Work out the finished part from the listing and answer in its coordinate system (mm). Face numbers are marked on the shaded views. A direction names the side the tool comes from. Give positions to 0.01 mm unless a question says otherwise; leave off trailing zeros. Loops run counter-clockwise (first coordinate to the right, second up) from the corner with the lowest first, then second, coordinate; pieces in that order, holes last.
from build123d import *

# Parameters (mm, degrees)
SHIM_TOP_START          = -1.6
SHIM_SKETCH_W           = 10.2
SHIM_SKETCH_H           = 2.6
SHIM_TOP_DEPTH          = 8.4
SHIM_BOTTOM_OUTLINE_W   = 10.027211308
SHIM_BOTTOM_OUTLINE_H   = 2.427211308
SHIM_BOTTOM_DEPTH       = 19.8
SHIM_BOTTOM_DRAFT       = -0.25
CHAMFER_2_SIZE          = 1
CHAMFER_2_SIZE2         = 1.745257156
RETAINING_BUMP_SKETCH_R = 3.5
RETAINING_BUMP_DEPTH    = 0.3
FILLET1_R               = 0.3


# Read off the part's stored shape, not the designer's step: shim_bottom
with BuildPart() as part:
    # shim_sketch → shim_top (new body)
    with BuildSketch(Plane.XY.offset(SHIM_TOP_START)):
        with Locations((-242.85, 41.3)):
            Rectangle(SHIM_SKETCH_W, SHIM_SKETCH_H)
    extrude(amount=-SHIM_TOP_DEPTH)


with BuildPart() as shim_bottom_tool:
    # shim_bottom outline → shim_bottom (with draft: the straight prism first)
    with BuildSketch(Plane.XY.offset(-29.8)):
        with Locations((-242.85, 41.3)):
            Rectangle(SHIM_BOTTOM_OUTLINE_W, SHIM_BOTTOM_OUTLINE_H)
    extrude(amount=SHIM_BOTTOM_DEPTH)
    # shim_bottom: the draft: its side faces are tilted about the plane it starts from
    shim_bottom_sides = [shim_bottom_tool.faces().sort_by_distance(p)[0] for p in [
        (-242.85, 40.086394346, -19.9),
        (-237.836394346, 41.3, -19.9),
        (-242.85, 42.513605654, -19.9),
        (-247.863605654, 41.3, -19.9),
    ]]
    draft(shim_bottom_sides, Plane.XY.offset(-29.8), SHIM_BOTTOM_DRAFT)


with BuildPart() as part_1:
    add(part.part)

    # shim_bottom: add shim_bottom_tool
    add(shim_bottom_tool.part)

    # Chamfer 2
    chamfer_2_edges = [part_1.edges().sort_by_distance(p)[0] for p in [
        (-237.836394346, 41.3, -29.8),
        (-242.85, 42.513605654, -29.8),
        (-247.863605654, 41.3, -29.8),
        (-242.85, 40.086394346, -29.8),
    ]]
    chamfer_2_side = [part_1.faces().sort_by_distance(p)[0] for p in [
        (-242.85, 41.3, -29.8),
    ]]
    chamfer(chamfer_2_edges, length=CHAMFER_2_SIZE, length2=CHAMFER_2_SIZE2, reference=chamfer_2_side[0])

    # retaining_bump_sketch → retaining_bump (add)
    with BuildSketch(Plane(origin=(0, 42.642821639, -0.186065591), x_dir=(1, 0, 0), z_dir=(0, 0.9999904807207346, -0.004363309284746581))):
        with Locations(Location((-242.85, 14.618579624, 0), (0, 0, 270))):
            Circle(RETAINING_BUMP_SKETCH_R)
    extrude(amount=RETAINING_BUMP_DEPTH)

    # Fillet1
    fillet1_edges = [part_1.edges().sort_by_distance(p)[0] for p in [
        (-242.85, 42.863761816, -18.305781732),
    ]]
    fillet(fillet1_edges, radius=FILLET1_R - 0.0001)  # a hair under: the kernel refuses the full size


solid = part_1.part
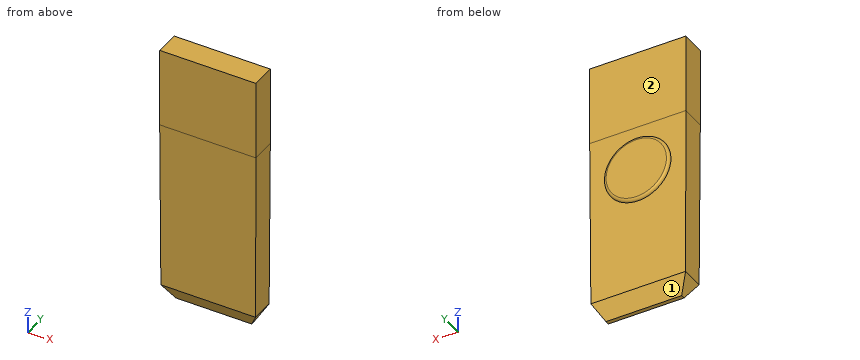
Item 1: Find section C-C, the plane z = -7. Write down the section's boundary in (x, y), plus the area to 3 significant figures.
Item 2: Flat-ended cylindrical pins translate along their axes: pin 1 Ø1 at (x, z) = (-240, -15) entering from -Y; pin 2 Ø1.5 at (y, z) = (40.5, -26) entering from +X; pin 3 Ø2 at (x, z) = (-246, -26.5) entering from -Y. Find the tip coordinate at first contact, or state that the pin passes through.
Item 3: Find section A-A, the plane x = -238.25. Write down the section's boundary in (y, z).
Item 4: For the marked faces 1 and 2, determine the directions among +Z, -Z, +X, -X, +Y, -Y from which every point of the face is accessible in a straight line to the end or side of a thin tool.
Item 5: Find section D-D, the plane z = -19.25. Write down the section's boundary in (x, y), plus the area to 3 significant figures.
Item 6: Consider line 1 (Y direction, x = -238.75, z = -3.5); line 2 (X direction, y = 41.95, z = -26.75); line 3 (Y direction, x = -246, z = -27.75). Determine where each line is inside the solid, lowest interval first.
Item 7: Find section B-B, the plane y = 40.6. Write down the section's boundary in (x, z), plus the area to 3 significant figures.
Ans:
1. outline: (-247.95, 40) - (-237.75, 40) - (-237.75, 42.6) - (-247.95, 42.6) - close
1. area: 26.5 mm2
2. pin 1: stops at y = 40.02
2. pin 2: stops at x = -237.82
2. pin 3: stops at y = 40.07
3. outline: (40, -10) - (40.08, -28.05) - (40.5, -28.78) - (42.1, -28.78) - (42.52, -28.05) - (42.6, -10) - (42.6, -1.6) - (40, -1.6) - close
4. face 1: -Z, +X, -X, +Y
4. face 2: +Z, +X, -X, +Y
5. outline: (-247.91, 40.04) - (-237.79, 40.04) - (-237.79, 42.56) - (-247.91, 42.56) - close
5. area: 25.5 mm2
6. line 1: y = 40 to 42.6
6. line 2: x = -247.88 to -237.82
6. line 3: y = 40.08 to 42.52
7. outline: (-247.95, -10) - (-247.87, -28.05) - (-247.35, -28.96) - (-238.35, -28.96) - (-237.83, -28.05) - (-237.75, -10) - (-237.75, -1.6) - (-247.95, -1.6) - close
7. area: 277 mm2
